The listing builds one solid part. Answer for the finished solid, in the listing's coordinates (mm). A direction names the side the tool comes from. Coordinates: 2 decimals unless noted, no trailing zeros. Order: outer loops, then holes, each group sorted by start corner. A loop starts at its lowest first (then second) coordinate and runs counter-clockwise, first axis right, second up. Notation, with made-up numbers: (88, 49) -> (140, 49) arc R17 cw to (140, 68) -> close; hole circle Ø2 at (-33, -29.75). An arc over 180 degrees is marked (long way). Return JSON: item names as keys, results as strings.
```python
from build123d import *

# Parameters (mm, degrees)
CROQUIS1_W              = 40.35
CROQUIS1_H              = 29.9
CROQUIS1_R              = 2
SALIENTE_EXTRUIR1_DEPTH = 2.05
CORTAR_EXTRUIR2_DEPTH   = 1.65
CROQUIS3_W              = 13
CROQUIS3_H              = 13
CORTAR_EXTRUIR3_DEPTH   = 47.737063506
REDONDEO2_R             = 0.5
CHAFL_N1_SIZE           = 0.4
REDONDEO4_R             = 1.27
SALIENTE_EXTRUIR3_START = -2.05
SALIENTE_EXTRUIR3_DEPTH = 4.25
SALIENTE_EXTRUIR4_DEPTH = 1.65
CROQUIS9_R              = 0.25
CROQUIS11_R             = 0.25
REDONDEO6_R             = 1.5
REDONDEO7_R             = 0.5
REDONDEO8_R             = 0.5
CHAFL_N2_SIZE           = 0.4


# Some blends are built 0.0001 mm under size
with BuildPart() as part:
    # Croquis1 → Saliente-Extruir1 (new body)
    with BuildSketch(Plane(origin=(0, 0, 0), x_dir=(1, 0, 0), z_dir=(0, 1, 0))):
        with Locations((14.905897563, 15.863653327)):
            Rectangle(CROQUIS1_W, CROQUIS1_H)
        with Locations(Location((3.230897563, 3.913653327, 0), (0, 0, 270))):
            Circle(CROQUIS1_R, mode=Mode.SUBTRACT)
        with Locations(Location((30.580897563, 27.413653327, 0), (0, 0, 270))):
            Circle(CROQUIS1_R, mode=Mode.SUBTRACT)
    extrude(amount=SALIENTE_EXTRUIR1_DEPTH)

    # Croquis2 → Cortar-Extruir2 (cut)
    with BuildSketch(Plane(origin=(0, 2.05, 0), x_dir=(1, 0, 0), z_dir=(0, 1, 0))):
        with BuildLine():
            Line((27.580897563, 27.413653327), (27.580897563, 29.313653327))
            Line((27.580897563, 29.313653327), (22.880897563, 29.313653327))
            Line((22.880897563, 29.313653327), (22.880897563, 26.613653327))
            Line((22.880897563, 26.613653327), (22.880897563, 11.713653327))
            Line((22.880897563, 11.713653327), (7.980897563, 11.713653327))
            Line((7.980897563, 11.713653327), (7.980897563, 26.613653327))
            Line((7.980897563, 26.613653327), (7.980897563, 29.313653327))
            Line((7.980897563, 29.313653327), (3.230897563, 29.313653327))
            Line((3.230897563, 29.313653327), (3.230897563, 2.413653327))
            Line((3.230897563, 2.413653327), (27.6, 2.413653327))
            Line((27.6, 2.413653327), (27.6, 0.913653327))
            Line((27.6, 0.913653327), (32.580897563, 0.913653327))
            Line((32.580897563, 0.913653327), (32.580897563, 24.413653327))
            Line((32.580897563, 24.413653327), (30.580897563, 24.413653327))
            ThreePointArc((30.580897563, 24.413653327), (28.459577219, 25.292332983), (27.580897563, 27.413653327))
        make_face()
    extrude(amount=-CORTAR_EXTRUIR2_DEPTH, mode=Mode.SUBTRACT)

    # Croquis3 → Cortar-Extruir3 (cut, through all)
    with BuildSketch(Plane(origin=(0, 2.05, 0), x_dir=(1, 0, 0), z_dir=(0, 1, 0))):
        with Locations((15.580897563, 19.313653327)):
            Rectangle(CROQUIS3_W, CROQUIS3_H)
    extrude(amount=-CORTAR_EXTRUIR3_DEPTH, mode=Mode.SUBTRACT)

    # Redondeo2
    redondeo2_edges = [part.edges().sort_by_distance(p)[0] for p in [
        (9.080897563, 1.025, -12.813653327),
        (9.080897563, 1.025, -25.813653327),
        (22.080897563, 1.025, -25.813653327),
        (22.080897563, 1.025, -12.813653327),
    ]]
    fillet(redondeo2_edges, radius=REDONDEO2_R)

    # Chaflán1
    chafl_n1_edges = [part.edges().sort_by_distance(p)[0] for p in [
        (15.580897563, 0, -25.813653327),
        (22.080897563, 0, -19.313653327),
        (15.580897563, 0, -12.813653327),
        (9.080897563, 0, -19.313653327),
        (21.934450953, 0, -25.667206717),
        (21.934450953, 0, -12.960099936),
        (9.227344172, 0, -12.960099936),
        (9.227344172, 0, -25.667206717),
    ]]
    chamfer(chafl_n1_edges, length=CHAFL_N1_SIZE)

    # Redondeo4
    redondeo4_edges = [part.edges().sort_by_distance(p)[0] for p in [
        (-5.269102437, 1.025, -30.813653327),
        (35.080897563, 1.025, -30.813653327),
        (35.080897563, 1.025, -0.913653327),
        (-5.269102437, 1.025, -0.913653327),
    ]]
    fillet(redondeo4_edges, radius=REDONDEO4_R)

    # Croquis6 → Saliente-Extruir3 (add)
    with BuildSketch(Plane(origin=(0, 2.05, 0), x_dir=(1, 0, 0), z_dir=(0, 1, 0)).offset(SALIENTE_EXTRUIR3_START)):
        with BuildLine():
            Line((-3.999102437, 30.813653327), (33.810897563, 30.813653327))
            ThreePointArc((33.810897563, 30.813653327), (34.708923175, 30.441678939), (35.080897563, 29.543653327))
            Line((35.080897563, 29.543653327), (35.880897563, 29.543653327))
            ThreePointArc((35.880897563, 29.543653327), (35.2746086, 31.007364364), (33.810897563, 31.613653327))
            Line((33.810897563, 31.613653327), (-3.999102437, 31.613653327))
            Line((-3.999102437, 31.613653327), (-3.999102437, 30.813653327))
        make_face()
        with BuildLine():
            Line((27.6, 0.913653327), (-3.999102437, 0.913653327))
            ThreePointArc((-3.999102437, 0.913653327), (-4.89712805, 1.285627715), (-5.269102437, 2.183653327))
            Line((-5.269102437, 2.183653327), (-6.069102437, 2.183653327))
            ThreePointArc((-6.069102437, 2.183653327), (-5.462813475, 0.71994229), (-3.999102437, 0.113653327))
            Line((-3.999102437, 0.113653327), (27.6, 0.113653327))
            Line((27.6, 0.113653327), (27.6, 0.913653327))
        make_face()
    extrude(amount=SALIENTE_EXTRUIR3_DEPTH)

    # Croquis7 → Saliente-Extruir4 (add)
    with BuildSketch(Plane(origin=(0, 0.4, 0), x_dir=(1, 0, 0), z_dir=(0, 1, 0))):
        with BuildLine():
            ThreePointArc((6.230897563, 3.913653327), (5.352217906, 6.03497367), (3.230897563, 6.913653327))
            Line((3.230897563, 6.913653327), (3.230897563, 5.913653327))
            ThreePointArc((3.230897563, 5.913653327), (5.101726256, 4.620760108), (4.553773218, 2.413653327))
            Line((4.553773218, 2.413653327), (6.230897563, 2.413653327))
            Line((6.230897563, 2.413653327), (6.230897563, 3.913653327))
        make_face()
    extrude(amount=SALIENTE_EXTRUIR4_DEPTH)

    # Barrer1: sweep along a path in Croquis10
    with BuildLine(Plane(origin=(0, 4.25, 0), x_dir=(1, 0, 0), z_dir=(0, 1, 0))) as barrer1_path:
        Line((-3.999102437, 30.813653327), (33.810897563, 30.813653327))
        ThreePointArc((33.810897563, 30.813653327), (34.708923175, 30.441678939), (35.080897563, 29.543653327))
    # Croquis9 → Barrer1 (sweep)
    with BuildSketch(Plane.XY.offset(-29.543653327)):
        with Locations((35.080897563, 4)):
            Circle(CROQUIS9_R)
    sweep(path=barrer1_path.line)

    # Barrer2: sweep along a path in Croquis12
    with BuildLine(Plane(origin=(0, 4.25, 0), x_dir=(1, 0, 0), z_dir=(0, 1, 0))) as barrer2_path:
        Line((27.6, 0.913653327), (-3.999102437, 0.913653327))
        ThreePointArc((-3.999102437, 0.913653327), (-4.89712805, 1.285627715), (-5.269102437, 2.183653327))
    # Croquis11 → Barrer2 (sweep)
    with BuildSketch(Plane(origin=(0, 0, -2.183653327), x_dir=(-1, 0, 0), z_dir=(0, 0, -1))):
        with Locations((5.269102437, 4)):
            Circle(CROQUIS11_R)
    sweep(path=barrer2_path.line)

    # Redondeo6
    redondeo6_edges = [part.edges().sort_by_distance(p)[0] for p in [
        (3.230897563, 1.225, -6.913653327),
        (6.230897563, 1.225, -2.413653327),
        (3.230897563, 1.225, -29.313653327),
        (7.980897563, 1.225, -29.313653327),
        (22.880897563, 1.225, -29.313653327),
        (27.580897563, 1.225, -29.313653327),
        (32.580897563, 1.225, -24.413653327),
    ]]
    fillet(redondeo6_edges, radius=REDONDEO6_R - 0.0001)  # a hair under: the kernel refuses the full size

    # Redondeo7
    redondeo7_edges = [part.edges().sort_by_distance(p)[0] for p in [
        (7.980897563, 1.225, -11.713653327),
        (22.880897563, 1.225, -11.713653327),
    ]]
    fillet(redondeo7_edges, radius=REDONDEO7_R)

    # Redondeo8
    # the kernel refuses this fillet: 0.5 mm, written as the material it adds along each edge
    with BuildSketch(Plane(origin=(33.810897563, 2.05, -30.813653327), x_dir=(0, 0, 1), z_dir=(-1, 0, 0))) as redondeo8_piece_1:
        with BuildLine():
            CenterArc((REDONDEO8_R, REDONDEO8_R), REDONDEO8_R, 180, 90)
            Line((0, REDONDEO8_R), (0, 0))
            Line((0, 0), (REDONDEO8_R, 0))
        make_face()
    extrude(amount=37.81)
    with BuildSketch(Plane(origin=(-3.999102437, 2.05, -0.913653327), x_dir=(0, 0, -1), z_dir=(1, 0, 0))) as redondeo8_piece_2:
        with BuildLine():
            CenterArc((REDONDEO8_R, REDONDEO8_R), REDONDEO8_R, 180, 90)
            Line((0, REDONDEO8_R), (0, 0))
            Line((0, 0), (REDONDEO8_R, 0))
        make_face()
    extrude(amount=31.599102437)
    with BuildSketch(Plane(origin=(33.810897563, 2.05, -29.543653327), x_dir=(1, 0, 0), z_dir=(0, 0, 1))) as redondeo8_piece_3:
        with BuildLine():
            CenterArc((1.27 - REDONDEO8_R, REDONDEO8_R), REDONDEO8_R, 270, 90)
            Line((1.27, REDONDEO8_R), (1.27, 0))
            Line((1.27, 0), (1.27 - REDONDEO8_R, 0))
        make_face()
    revolve(axis=Axis((33.810897563, 2.05, -29.543653327), (0, 1, 0)), revolution_arc=90)
    with BuildSketch(Plane(origin=(-3.999102437, 2.05, -2.183653327), x_dir=(0, 0, 1), z_dir=(1, 0, 0))) as redondeo8_piece_4:
        with BuildLine():
            CenterArc((1.27 - REDONDEO8_R, -REDONDEO8_R), REDONDEO8_R, 0, 90)
            Line((1.27, -REDONDEO8_R), (1.27, 0))
            Line((1.27, 0), (1.27 - REDONDEO8_R, 0))
        make_face()
    revolve(axis=Axis((-3.999102437, 2.05, -2.183653327), (0, -1, 0)), revolution_arc=90)

    # Chaflán2
    chafl_n2_edges = [part.edges().sort_by_distance(p)[0] for p in [
        (-5.269102437, 0, -15.863653327),
        (-5.669102437, 0, -2.183653327),
        (-5.462813475, 0, -0.71994229),
        (11.800448781, 0, -0.113653327),
        (27.6, 0, -0.513653327),
        (30.705448781, 0, -0.913653327),
        (34.708923175, 0, -1.285627715),
        (35.080897563, 0, -15.863653327),
        (35.480897563, 0, -29.543653327),
        (35.2746086, 0, -31.007364364),
        (14.905897563, 0, -31.613653327),
        (-3.999102437, 0, -31.213653327),
        (-4.89712805, 0, -30.441678939),
    ]]
    chamfer(chafl_n2_edges, length=CHAFL_N2_SIZE - 0.0001)  # a hair under: the kernel refuses the full size


solid = part.part
```
Item 1: The part is cut by section B-B on y = 3.1. Determine the outline of the cut face in (x, z).
Answer list:
{"outline": "(-6.07, -2.18) -> (-5.27, -2.18) arc R1.27 cw to (-4, -0.91) -> (27.6, -0.91) -> (27.6, -0.11) -> (-4, -0.11) arc R2.07 ccw to start; (-4, -31.61) -> (33.81, -31.61) arc R2.07 ccw to (35.88, -29.54) -> (35.08, -29.54) arc R1.27 cw to (33.81, -30.81) -> (-4, -30.81) -> close"}
Item 2: Determine the mould class of faces 1 (the flat face through (16, 4.25, -31)), 2 (the cylindrical face through (7.53, 1.213, -28.886)), 3 (the cylindrical face through (-4.89, 3.14, -1.28)) for opening direction X: pulls with the +X half, pulls with the -X half, needs draft (parallel to the pull), parting line crosses it, or undercut.
Answer list:
{"face 1": "needs draft", "face 2": "undercut", "face 3": "pulls with the +X half"}
Item 3: The part is cut by section A-A on z = -16. Determine the outline of the cut face in (x, y), plus the area to 3 significant figures.
Answer list:
{"outline": "(-5.27, 0.4) -> (-4.87, 0) -> (8.68, 0) -> (9.08, 0.4) -> (9.08, 2.05) -> (7.98, 2.05) -> (7.98, 0.4) -> (3.23, 0.4) -> (3.23, 2.05) -> (-5.27, 2.05) -> close; (22.08, 0.4) -> (22.48, 0) -> (34.68, 0) -> (35.08, 0.4) -> (35.08, 2.05) -> (32.58, 2.05) -> (32.58, 0.4) -> (22.88, 0.4) -> (22.88, 2.05) -> (22.08, 2.05) -> close", "area": "31.9 mm2"}
Item 4: The part is cut by section C-C on x = 0. Determine the outline of the cut face in (y, z).
Answer list:
{"outline": "(0, -31.21) -> (0.4, -31.61) -> (4.25, -31.61) -> (4.25, -30.81) arc R0.25 ccw to (3.75, -30.81) -> (2.55, -30.81) arc R0.5 cw to (2.05, -30.31) -> (2.05, -1.41) arc R0.5 cw to (2.55, -0.91) -> (3.75, -0.91) arc R0.25 ccw to (4.25, -0.91) -> (4.25, -0.11) -> (0.4, -0.11) -> (0, -0.51) -> close"}
Item 5: Which of the six approach directions +Z, -Z, +X, -X, +Y, -Y give full straight-line access (tool end or side, diameter ignored) to faces 4 (the flat face through (15, 3, -30.814)), 5 (the conical face through (9.124, 0.247, -12.847)), 6 (the flat face through (25, 1, -29.314))?
Answer list:
{"face 4": "-X", "face 5": "-Y", "face 6": "+Y"}
Item 6: Find the intervals of material crossed by probe 1 along X at (y, z) = (0.9, -18); probe 2 along Z at (x, y) = (20.5, 1.6); probe 3 along X at (y, z) = (1.8, -5), in increasing order.
Answer list:
{"probe 1": "-5.27 to 3.23, 7.98 to 9.08, 22.08 to 22.88, 32.58 to 35.08", "probe 2": "-31.61 to -25.81, -12.81 to -11.71, -2.41 to -0.11", "probe 3": "-5.27 to 1.55, 4.91 to 6.03, 32.58 to 35.08"}
Item 7: Flat-ended cylindrical pins translate along their axes: pin 1 (1 mm diameter, centred on x = 20.5, z = -25.5, fed in from -Y); pin 2 (1.3 mm diameter, centred on y = 1, z = -19, fed in from -X); pin 3 (3 mm diameter, centred on x = 0, z = -11.5, fed in from +Y); pin 4 (2.5 mm diameter, centred on x = 3.23, z = -3.91, fed in from -Y). Find the tip coordinate at first contact, or state that the pin passes through.
Answer list:
{"pin 1": "y = 0.21", "pin 2": "x = -5.27", "pin 3": "y = 2.05", "pin 4": "through"}
